Autodesk Inventor part; units mm, degrees
ref_plane "YZ Plane" through (0, 0, 0) normal (1, 0, 0) x (0, 1, 0)
ref_plane "XZ Plane" through (0, 0, 0) normal (0, 1, 0) x (-1, 0, 0)
ref_plane "XY Plane" through (0, 0, 0) normal (0, 0, 1) x (1, 0, 0)
sketch "Sketch1" plane through (0, 0, 0) normal (0, 0, 1) x (1, 0, 0)
  line L0 (-3.4184, -2.6565) -> (3.4184, -2.6565)
  line L1 (3.4184, -2.6565) -> (3.4184, 2.6565)
  line L2 (3.4184, 2.6565) -> (-3.4184, 2.6565)
  line L3 (-3.4184, 2.6565) -> (-3.4184, -2.6565)
  line L4 (-3.4184, -2.6565) -> (3.4184, 2.6565) construction
  line L5 (3.4184, -2.6565) -> (-3.4184, 2.6565) construction
  line L6 (-2.3603, -1.8342) -> (2.3603, -1.8342)
  line L7 (2.3603, -1.8342) -> (2.3603, 1.8342)
  line L8 (2.3603, 1.8342) -> (-2.3603, 1.8342)
  line L9 (-2.3603, 1.8342) -> (-2.3603, -1.8342)
  line L10 (-2.3603, -1.8342) -> (2.3603, 1.8342) construction
  line L11 (2.3603, -1.8342) -> (-2.3603, 1.8342) construction
  point P0 (0, 0)
extrude "Extrusion1" add sketch "Sketch1" along normal blind 10
sketch "Sketch2" plane through (3.4184, -2.6565, 0) normal (1, 0, 0) x (0, 0, -1)
  circle A0 centre (-4.8161, 2.6565) radius 1.0093
  circle A1 centre (-4.8161, 2.6565) radius 0.782
  point P0 (0, 2.6565)
extrude "Extrusion2" add sketch "Sketch2" along normal blind 2
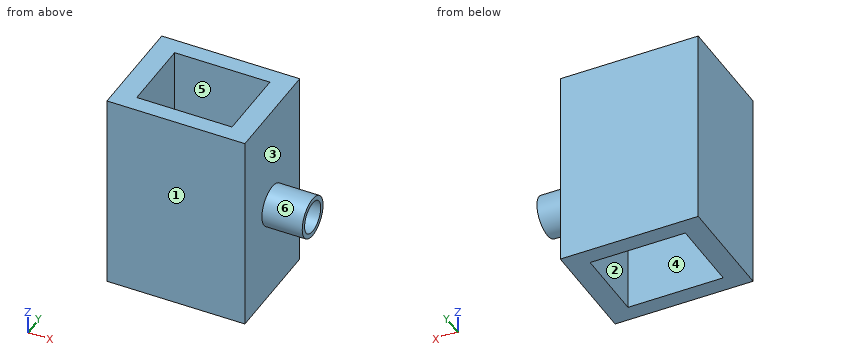
CAD build for the part. Positions are in the model's coordinates, mm. Face numbers are marked on the shaded views. A direction names the side the tool comes from. Round coordinates to 2 decimals unless told otherwise and drop trailing zeros. Write each loop counter-clockwise with the first axis right and the second up, starting at its lowest first coordinate (ties: lowest second). Pieces come first, ordered by that corner, then holes. Notation, with made-up numbers: M 20,22 L 64,22 A6 cw 64,29 Z; hole C 85.5,-15 d4. An arc over 180 degrees is marked long. Put each result on its own line as item: value. Start each with the question number.
1) 3-axis set-ups, long thin cutter, end or side, ignore diameter. For the marked faces 1 and 2: which of +Z, -Z, +X, -X, +Y, -Y reach the whole face in a straight line?
2) Saw through at D-D, the plane y = -1.25. Write the cut outline in (x, z).
3) Saw through at C-C, the plane x = 4.75. Write the cut outline in (y, z), and give its area (3 significant figures).
4) Pull direction X, two halves, no side cores. Call the marked faces 3, 4, 5 and 6: pulls with the +X half, pulls with the -X half, needs draft (parallel to the pull), parting line crosses it, or undercut.
5) Saw through at A-A, the plane y = 0. Write the cut outline in (x, z).
6) Saw through at B-B, the plane z = 1. Write the cut outline in (x, y).
7) Pin check, flat tips, straight feed: pin 1 Ø1.8 at (y, z) = (0, 4.82) entering from +X; pin 2 Ø0.8 at (y, z) = (0, 5) entering from +X. Stop position of each tip, or through.
8) Drill centre lines: probe 1 along X at (y, z) = (0.9, 1.5); probe 2 along Y at (x, z) = (-0.5, 3.75); probe 3 along X at (y, z) = (-2.1, 7.5). Where is each one in solid material? Low to high. Write a range as [from, to].
Resolved:
1. face 1: +Z, -Z, +X, -X, -Y
1. face 2: +Z, -Z
2. outline: M -3.42,0 L -2.36,0 L -2.36,10 L -3.42,10 Z; M 2.36,0 L 3.42,0 L 3.42,10 L 2.36,10 Z
3. outline: C 0,4.82 d2.02; hole C 0,4.82 d1.56
3. area: 1.28 mm²
4. face 3: pulls with the +X half
4. face 4: undercut
4. face 5: undercut
4. face 6: needs draft
5. outline: M -3.42,0 L -2.36,0 L -2.36,10 L -3.42,10 Z; M 2.36,0 L 3.42,0 L 3.42,3.81 L 5.42,3.81 L 5.42,4.03 L 3.42,4.03 L 3.42,5.6 L 5.42,5.6 L 5.42,5.83 L 3.42,5.83 L 3.42,10 L 2.36,10 Z
6. outline: M -3.42,-2.66 L 3.42,-2.66 L 3.42,2.66 L -3.42,2.66 Z; hole M -2.36,-1.83 L 2.36,-1.83 L 2.36,1.83 L -2.36,1.83 Z
7. pin 1: x = 5.42
7. pin 2: x = 3.42
8. probe 1: [-3.42, -2.36], [2.36, 3.42]
8. probe 2: [-2.66, -1.83], [1.83, 2.66]
8. probe 3: [-3.42, 3.42]
